Geometry: final body of the model. Coordinates: model frame, mm. A direction names the side the tool comes from. Give positions to 0.01 mm unless a question says otherwise; leave off trailing zeros. Write each loop counter-clockwise with the first axis right and the second up, starting at its lowest first coordinate (ties: lowest second). Pieces come first, ordered by that corner, then holes.
Q1. Mould query, pull axis X, two halves, no side actions, for faces 1 (the cylindrical face through (18.5, -20.45, -23.55)), 2 (the flat face through (-5, -26, -24)), 3 (the cylindrical face through (38.58, -33.02, -28.03)). Classes: +X half, -X half, draft (parallel to the pull), parting line (faces both ways), or undercut.
Q2. Line query: line 1 (X direction, y = -1, z = -18); line 2 (Z direction, x = 9.5, y = -5.5); line 3 (Y direction, x = 4, z = 0). Output: solid intervals per line, ascending.
Q3. Section D-D (z = -26). State how many separate pieces and enclosed holes the cut face has, plus the area to 3 significant figures.
Q4. Pin query (flat end, axial travel): pin 1 Ø2.5 at (y, z) = (-34.11, -35.16) entering from +X; pin 2 Ø8 at (y, z) = (-29, -5.5) entering from +X; pin 3 Ø16.5 at (x, y) = (43.5, -21.5) entering from +Z; pin 4 Ø6 at (x, z) = (11.5, 14.5) entering from +Y. Return the tip coordinate at first contact, or that it passes through.
Q5. Section C-C (x = 11). Return the cut outline in (y, z).
Q6. Section B-B (z = 0). Return the cut outline in (x, y).
Q7. Section A-A (y = 0). Return the cut outline in (x, z), plus the area to 3 significant figures.
Q8. Reachability of faces 4 (the flat face through (-2, -5.098, -36)), 5 (the flat face through (0, -16, 4)), 6 (the flat face through (0, -22, -36)) from +Z, -Z, +X, -X, +Y, -Y: full face, straight path, thin tool, end or side. Return the list, or none.
from build123d import *

# Parameters (mm, degrees)
SKETCH1_R                             = 21.14
SKETCH1_R_2                           = 16.14
BOSS_EXTRUDE1_DEPTH                   = 17
BOSS_EXTRUDE2_DEPTH                   = 17
SKETCH3_W                             = 6
SKETCH3_H                             = 34.909785338
BOSS_EXTRUDE3_DEPTH                   = 60
CUT_EXTRUDE1_DEPTH                    = 30
FILLET1_R                             = 5
BOSS_EXTRUDE4_DEPTH                   = 5
FILLET2_R                             = 5
TAP_DRILL_FOR_M4X0_7_TAP1_D           = 3.3
TAP_DRILL_FOR_M4X0_7_TAP1_DEPTH       = 5
TAP_DRILL_FOR_M4X0_7_TAP1_CSINK_D     = 3.35
TAP_DRILL_FOR_M4X0_7_TAP1_CSINK_ANGLE = 100
TAP_DRILL_FOR_M4X0_7_TAP1_TIP         = 0.991420021
TAP_DRILL_FOR_M4X0_7_TAP2_D           = 3.3
TAP_DRILL_FOR_M4X0_7_TAP2_DEPTH       = 7
TAP_DRILL_FOR_M4X0_7_TAP2_CSINK_D     = 3.35
TAP_DRILL_FOR_M4X0_7_TAP2_CSINK_ANGLE = 100
TAP_DRILL_FOR_M4X0_7_TAP2_TIP         = 0.991420021


with BuildPart() as part:
    # Sketch1 → Boss-Extrude1 (new body)
    with BuildSketch(Plane(origin=(0, 0, 0), x_dir=(0, 0, -1), z_dir=(1, 0, 0))):
        Circle(SKETCH1_R)
        Circle(SKETCH1_R_2, mode=Mode.SUBTRACT)
    extrude(amount=BOSS_EXTRUDE1_DEPTH)

    # Sketch2 → Boss-Extrude2 (add)
    with BuildSketch(Plane.ZY):
        with BuildLine():
            Line((-30.978599342, -40.052160935), (-30.978599342, -5.142375597))
            Line((-30.978599342, -5.142375597), (-16.599116733, 13.09079538))
            ThreePointArc((-16.599116733, 13.09079538), (-13.09079538, -16.599116733), (16.599116733, -13.09079538))
            Line((16.599116733, -13.09079538), (-4.663804983, -40.052160935))
            Line((-4.663804983, -40.052160935), (-30.978599342, -40.052160935))
        make_face()
    extrude(amount=-BOSS_EXTRUDE2_DEPTH)

    # Sketch3 → Boss-Extrude3 (add)
    with BuildSketch(Plane(origin=(17, 0, 0), x_dir=(0, 0, -1), z_dir=(1, 0, 0))):
        with Locations((27.978599342, -22.597268266)):
            Rectangle(SKETCH3_W, SKETCH3_H)
    extrude(amount=BOSS_EXTRUDE3_DEPTH)

    # Sketch4 → Cut-Extrude1 (cut)
    with BuildSketch(Plane.XY.offset(-24.978599342)):
        Polygon((17, -5.142375597), (77, -22.597268266), (77, -5.142375597), align=None)
    extrude(amount=-CUT_EXTRUDE1_DEPTH, mode=Mode.SUBTRACT)

    # Fillet1
    fillet1_edges = [part.edges().sort_by_distance(p)[0] for p in [
        (17, -5.142375597, -27.978599342),
        (17, -22.597268266, -24.978599342),
        (77, -22.597268266, -27.978599342),
    ]]
    fillet(fillet1_edges, radius=FILLET1_R)

    # Sketch5 → Boss-Extrude4 (add)
    with BuildSketch(Plane.ZY):
        Polygon((-30.978599342, -5.098400642), (-41.06651396, -5.098400642), (-41.06651396, -39.736841718), (-25.501919328, -39.736841718), (-4.663804983, -39.736841718), align=None)
    extrude(amount=BOSS_EXTRUDE4_DEPTH)

    # Fillet2
    # the kernel refuses this fillet: 5 mm, written as the material it adds along each edge
    with BuildSketch(Plane(origin=(0, -49.690311531, 2.897837608), x_dir=(0, 0.604931407257239, 0.7962775850881252), z_dir=(0, 0.7962775850881253, -0.604931407257239))) as fillet2_piece_1_section:
        with BuildLine():
            CenterArc((FILLET2_R, -FILLET2_R), FILLET2_R, 90, 90)
            Line((0, -FILLET2_R), (0, 0))
            Line((0, 0), (FILLET2_R, 0))
        make_face()
    fillet2_piece_1 = extrude(amount=68.472330766, mode=Mode.PRIVATE)
    fillet2_piece_1 = split(fillet2_piece_1, bisect_by=Plane(origin=(-1.128828845, -8.634761076, -33.732848524), z_dir=(0, -0.6192429224168574, 0.7851994670379179)), keep=Keep.TOP, mode=Mode.PRIVATE)
    fillet2_piece_1 = split(fillet2_piece_1, bisect_by=Plane(origin=(-1.128828845, -34.816351836, -0.534615058), z_dir=(0, 0.6192429224168575, -0.7851994670379177)), keep=Keep.TOP, mode=Mode.PRIVATE)
    fillet2_piece_1 = split(fillet2_piece_1, bisect_by=Plane(origin=(-1.128828845, -39.736841718, -16.726060425), z_dir=(0, 1, 0)), keep=Keep.TOP, mode=Mode.PRIVATE)
    add(fillet2_piece_1)
    # the kernel refuses this fillet: 5 mm, written as the material it takes off along each edge
    with BuildSketch(Plane(origin=(-5, 7.401599358, -41.06651396), x_dir=(0, 0, 1), z_dir=(0, -1, 0))) as fillet2_2_piece_1:
        with BuildLine():
            CenterArc((FILLET2_R, -FILLET2_R), FILLET2_R, 90, 90)
            Line((0, -FILLET2_R), (0, 0))
            Line((0, 0), (FILLET2_R, 0))
        make_face()
    extrude(amount=59.638441075, mode=Mode.SUBTRACT)

    # Tap Drill for M4x0.7 Tap1
    with Locations(Plane.ZY.offset(5)):
        with Locations((-35.156261267, -14.70127854), (-35.156261267, -34.106690994)):
            CounterSinkHole(TAP_DRILL_FOR_M4X0_7_TAP1_D / 2, TAP_DRILL_FOR_M4X0_7_TAP1_CSINK_D / 2, depth=TAP_DRILL_FOR_M4X0_7_TAP1_DEPTH, counter_sink_angle=TAP_DRILL_FOR_M4X0_7_TAP1_CSINK_ANGLE)
            with Locations((0, 0, -(TAP_DRILL_FOR_M4X0_7_TAP1_DEPTH + TAP_DRILL_FOR_M4X0_7_TAP1_TIP / 2))):  # 118° drill point
                Cone(0, TAP_DRILL_FOR_M4X0_7_TAP1_D / 2, TAP_DRILL_FOR_M4X0_7_TAP1_TIP, mode=Mode.SUBTRACT)

    # Tap Drill for M4x0.7 Tap2
    with Locations(Plane.XY.offset(-24.978599342)):
        with Locations((36.93257039, -33.095127913), (63.418354043, -33.095127913)):
            CounterSinkHole(TAP_DRILL_FOR_M4X0_7_TAP2_D / 2, TAP_DRILL_FOR_M4X0_7_TAP2_CSINK_D / 2, depth=TAP_DRILL_FOR_M4X0_7_TAP2_DEPTH, counter_sink_angle=TAP_DRILL_FOR_M4X0_7_TAP2_CSINK_ANGLE)
            with Locations((0, 0, -(TAP_DRILL_FOR_M4X0_7_TAP2_DEPTH + TAP_DRILL_FOR_M4X0_7_TAP2_TIP / 2))):  # 118° drill point
                Cone(0, TAP_DRILL_FOR_M4X0_7_TAP2_D / 2, TAP_DRILL_FOR_M4X0_7_TAP2_TIP, mode=Mode.SUBTRACT)


solid = part.part
Computed:
1. face 1: +X half
1. face 2: -X half
1. face 3: undercut
2. line 1: x = 0 to 17
2. line 2: z = -30.98 to -15.17, 15.17 to 20.41
2. line 3: y = -34.14 to -16.14, 16.14 to 21.14
3. separate pieces: 1
3. enclosed holes: 2
3. area: 2,400 mm2
4. pin 1: passes through
4. pin 2: stops at x = 17
4. pin 3: stops at z = -24.98
4. pin 4: stops at y = 17.74
5. outline: (-40.05, -30.98) - (-5.14, -30.98) - (13.09, -16.6) arc R21.14 ccw to (-13.09, 16.6) - (-40.05, -4.66) - close; hole circle Ø32.28 at (0, 0)
6. outline: (0, -34.14) - (17, -34.14) - (17, -16.14) - (0, -16.14) - close; (0, 16.14) - (17, 16.14) - (17, 21.14) - (0, 21.14) - close
7. outline: (0, -26.92) - (17, -26.92) - (17, -16.14) - (0, -16.14) - close; (0, 16.14) - (17, 16.14) - (17, 21.14) - (0, 21.14) - close
7. area: 268 mm2
8. face 4: -Z, +X, -X, +Y
8. face 5: +Z, -X, +Y
8. face 6: -Z, +X, +Y, -Y
